from build123d import *

# Parameters (mm, degrees)
F0_W     = 26.5945848078
F0_H     = 6.6253300756
F1_DEPTH = 152.4
F2_DEPTH = 76.2
F3_DEPTH = 18.796
F4_SIZE2 = 24.9431344672
F4_SIZE  = 18.796
F6_R     = 5.08


with BuildPart() as f1:
    # F0 (on Top) → F1 (new body)
    with BuildSketch(Plane.XY):
        with Locations((-13.2972924039, 3.3126650378)):
            Rectangle(F0_W, F0_H)
    extrude(amount=F1_DEPTH)

    # F2 (add): a face of the model
    f2_faces = [f1.faces().sort_by_distance(p)[0] for p in [
        (-26.5945848078, 3.3126650378, 76.2),
    ]]
    extrude(f2_faces, amount=F2_DEPTH)

    # F3 (add): a face of the model
    f3_faces = [f1.faces().sort_by_distance(p)[0] for p in [
        (-51.3972924039, 6.6253300756, 76.2),
    ]]
    extrude(f3_faces, amount=F3_DEPTH)

    # F4
    f4_edges = [f1.edges().sort_by_distance(p)[0] for p in [
        (0, 25.42133, 76.2),
    ]]
    f4_side = f1.faces().sort_by_distance((-51.397292, 25.42133, 76.2))[0]
    chamfer(f4_edges, length=F4_SIZE, length2=F4_SIZE2, reference=f4_side)

    # F5: F1 across plane


with BuildPart() as f1_1:
    add(f1.part)
    add(f1.part.mirror(Plane.YZ))

    # F6
    f6_edges = [f1_1.edges().sort_by_distance(p)[0] for p in [
        (0, 0.478196, 76.2),
    ]]
    fillet(f6_edges, radius=F6_R)


solid = f1_1.part
Input: part model. Units: mm. Frame: model coordinates. A direction names the side the tool comes from. Give positions to 0.01 mm unless a question says otherwise; leave off trailing zeros. Write each loop counter-clockwise with the first axis right and the second up, starting at its lowest first coordinate (ties: lowest second). Pieces come first, ordered by that corner, then holes. Notation, with made-up numbers: M -14.5,64.5 L 20.5,64.5 A23 ccw 20.5,73.5 Z; hole C 77.25,23.5 d11. An arc over 180 degrees is marked long. Write item = value, one per line. Start each with the question number.
1) Reachability of faces 1 (the flat face through (11.32, 15.5, 75.13)), 2 (the flat face through (-102.795, 13, 75)) from +Z, -Z, +X, -X, +Y, -Y: full face, straight path, thin tool, end or side. Return the list, or none.
2) Material intervals for line 1 along X through (y, z) = (19.75, 94); line 2 along X through (y, z) = (6.5, 51); line 3 along Y through (x, z) = (9, 64), sorted ascending. Write a range as [from, to].
3) Draft query along X for faces 3 (the flat face through (102.795, 13, 75)), 4 (the flat face through (1, 1, 0)), 5 (the flat face through (-11.32, 15.5, 75.13)). Return one class per face: +X half, -X half, draft (parallel to the pull), parting line (faces both ways), or undercut.
4) Cut plane A-A on y = 17.5. Return the cut outline in (x, z).
5) Cut plane B-B on z = 20. Return the cut outline in (x, y).
6) Cut plane C-C on x = -8. Return the cut outline in (y, z).
Solved:
q1.face_1 = +Z, -Z, +Y
q1.face_2 = +Z, -Z, -X, +Y, -Y
q2.line_1 = [-102.79, -14.52], [14.52, 102.79]
q2.line_2 = [-102.79, -4.54], [4.54, 102.79]
q2.line_3 = [0, 12.42]
q3.face_3 = +X half
q3.face_4 = draft
q3.face_5 = undercut
q4.outline = M -102.79,0 L -12.83,0 L -12.83,152.4 L -102.79,152.4 Z; M 12.83,0 L 102.79,0 L 102.79,152.4 L 12.83,152.4 Z
q5.outline = M -102.79,0 L 102.79,0 L 102.79,25.42 L 18.8,25.42 L 4.06,5.86 A5.08 cw -4.06,5.86 L -18.8,25.42 L -102.79,25.42 Z
q6.outline = M 0,0 L 11.09,0 L 11.09,152.4 L 0,152.4 Z
